Verification items for the finished model (mm, model axes). A direction names the side the tool comes from. Coordinates: 2 decimals unless noted, no trailing zeros. Order: outer loops, then holes, each group sorted by start corner. A loop starts at its lowest first (then second) coordinate and runs counter-clockwise, first axis right, second up. Notation, with made-up numbers: M 24,41 L 53,41 A32 ccw 53,69 Z; hole C 30.25,49.5 d6. An arc over 180 degrees is marked long. Return JSON: item names as keys, results as strings. Group by question number.
1. Mould release check, pull along X, two halves, no side actions. Record for faces 1 (the conical face through (22.134, -7.162, -1.59)), 2 (the conical face through (9.24, 0.28, -6.41)), 3 (the cylindrical face through (38, 0, -6)): +X half, -X half, draft (parallel to the pull), parting line (faces both ways), or undercut.
2. Set-up check for faces 4 (the flat face through (48, 0, 0)), 5 (the flat face through (30.5, -6, -2)): record each of +Z, -Z, +X, -X, +Y, -Y from which the full face is reachable in a straight line by a thin tool's end or side.
3. Section check A-A, the plane y = 24. Record the cut outline in (x, z).
4. Gauge pin test, flat ends, axial feed: pin 1 (10 mm diameter, centred on x = 1, y = 9.5, fed in from -Z); pin 2 (3 mm diameter, centred on x = 21.5, z = -4.5, fed in from -Y). Record the tip position at first contact, or that the pin passes through.
5. Material ranges on line 1 along Z through (x, y) = (3.5, 1); line 2 along Z through (x, y) = (2.5, 7), recorded low to high.
```python
from build123d import *

# Parameters (mm, degrees)
F2_SIZE  = 1.5
F3_R     = 1
F4_DEPTH = 50
F5_R     = 1
F6_DEPTH = 50


with BuildPart() as f1:
    # F0 (on Front) → F1 (revolve)
    with BuildSketch(Plane.XZ):
        with BuildLine():
            ThreePointArc((8.9969651904, 6.328871729), (-3.3191401677, 10.4872927177), (-11, 0))
            Line((-11, 0), (48, 0))
            Line((48, 0), (48, 6))
            Line((48, 6), (30.5, 6))
            Line((30.5, 6), (30.5, 6.5))
            Line((30.5, 6.5), (14, 8.1498274807))
            Line((14, 8.1498274807), (8.9969651904, 6.328871729))
        make_face()
    revolve(axis=Axis((18.5, 0, 0), (-1, 0, 0)))

    # F2
    f2_edges = [f1.edges().sort_by_distance(p)[0] for p in [
        (48, 0, -6),
    ]]
    chamfer(f2_edges, length=F2_SIZE)

    # F3 (on Front) → F4 (join, symmetric)
    with BuildSketch(Plane.XZ):
        Circle(F3_R)
    extrude(amount=F4_DEPTH, both=True)

    # F5 (on Top) → F6 (join, symmetric)
    with BuildSketch(Plane.XY):
        Circle(F5_R)
    extrude(amount=F6_DEPTH, both=True)


solid = f1.part
```
Answers follow:
{
 "1": {"face 1": "+X half", "face 2": "undercut", "face 3": "draft"},
 "2": {"face 4": "+Z, -Z, +X, +Y, -Y", "face 5": "+X"},
 "3": {"outline": "C 0,0 d2"},
 "4": {"pin 1": "z = -10.01", "pin 2": "y = -6.78"},
 "5": {"line 1": "-10.38 to 10.38", "line 2": "-8.11 to 8.11"}
}
